```python
from build123d import *

# Parameters (mm, degrees)
SKETCH4_R             = 1.5
BOSS_EXTRUDE3_DEPTH   = 15
BOSS_EXTRUDE3_2_DEPTH = 15
BOSS_EXTRUDE3_3_DEPTH = 15
BOSS_EXTRUDE23_START  = 15
BOSS_EXTRUDE23_DEPTH  = 4
BOSS_EXTRUDE24_START  = 8
BOSS_EXTRUDE24_DEPTH  = 4
FILLET2_R             = 2
FILLET1_R             = 1.5


# Read off the part's stored shape, not the designer's step: Mirror15
with BuildPart() as part:
    # Sketch4 → Boss-Extrude3 (new, symmetric)
    with BuildSketch(Plane.XY):
        with BuildLine():
            ThreePointArc((-15.745615363, 108.217071894), (-14.863780591, 107.808507644), (-13.893474834, 107.863861505))
            ThreePointArc((-13.893474834, 107.863861505), (-10.727575159, 106.958592694), (-10.299299114, 103.693778456))
            ThreePointArc((-10.299299114, 103.693778456), (-11.193367854, 101.14903756), (-11.496495568, 98.468892279))
            Line((-11.496495568, 98.468892279), (-11.496495568, 91.5))
            Line((-11.496495568, 91.5), (-13, 90))
            Line((-13, 90), (-14.503504432, 90))
            Line((-14.503504432, 90), (-14.503504432, 95.734709942))
            ThreePointArc((-14.503504432, 95.734709942), (-17.04172216, 103.115406131), (-23.582617138, 107.373800002))
            ThreePointArc((-23.582617138, 107.373800002), (-29.032421023, 126.907705171), (-20.414545428, 145.265429262))
            ThreePointArc((-20.414545428, 145.265429262), (-19.127581616, 145.281958408), (-19.054880744, 143.996943368))
            ThreePointArc((-19.054880744, 143.996943368), (-24.95633052, 125.408148717), (-15.745615363, 108.217071894))
        make_face()
        with Locations((-13, 105)):
            Circle(SKETCH4_R, mode=Mode.SUBTRACT)
    extrude(amount=BOSS_EXTRUDE3_DEPTH, both=True)



with BuildPart() as body_2:
    # Sketch4 → Boss-Extrude3 2 (new, symmetric)
    with BuildSketch(Plane.XY):
        with BuildLine():
            ThreePointArc((-15.463298435, 144.692144482), (-19.624699769, 139.278232713), (-21.960734627, 132.861797344))
            ThreePointArc((-21.960734627, 132.861797344), (-20.98224362, 131.398279383), (-19.518725659, 132.37677039))
            ThreePointArc((-19.518725659, 132.37677039), (-17.442455247, 138.079705369), (-13.743797057, 142.891596244))
            ThreePointArc((-13.743797057, 142.891596244), (-13.703273627, 144.651621052), (-15.463298435, 144.692144482))
        make_face()
    extrude(amount=BOSS_EXTRUDE3_2_DEPTH, both=True)


with BuildPart() as body_3:
    # Sketch4 → Boss-Extrude3 3 (new, symmetric)
    with BuildSketch(Plane.XY):
        with BuildLine():
            ThreePointArc((-18.842097465, 122.098018813), (-15.492555186, 116.010374953), (-10.254266127, 111.445381089))
            ThreePointArc((-10.254266127, 111.445381089), (-9.828866365, 109.737058954), (-11.5371885, 109.311659193))
            ThreePointArc((-11.5371885, 109.311659193), (-17.430845593, 114.447784397), (-21.199452745, 121.297059992))
            ThreePointArc((-21.199452745, 121.297059992), (-20.421254515, 122.876217042), (-18.842097465, 122.098018813))
        make_face()
    extrude(amount=BOSS_EXTRUDE3_3_DEPTH, both=True)


with BuildPart() as part_1:
    add(part.part)

    add(body_2.part)  # Boss-Extrude23 merges body 2

    add(body_3.part)  # Boss-Extrude23 merges body 3
    # Sketch81 → Boss-Extrude23 (add)
    with BuildSketch(Plane.XY.offset(BOSS_EXTRUDE23_START)):
        with BuildLine():
            ThreePointArc((-16.40923932, 143.732728133), (-16.959334589, 143.117801193), (-17.486399904, 142.483023987))
            ThreePointArc((-17.486399904, 142.483023987), (-20.86751312, 139.665952099), (-23.582500348, 136.202331891))
            ThreePointArc((-23.582500348, 136.202331891), (-23.172403472, 137.265482274), (-22.71440592, 138.308893232))
            ThreePointArc((-22.71440592, 138.308893232), (-19.828313947, 141.330604813), (-16.40923932, 143.732728133))
        make_face()
        with BuildLine():
            ThreePointArc((-14.984055873, 111.863377416), (-19.218265584, 114.528225057), (-23.012819409, 117.788793427))
            ThreePointArc((-23.012819409, 117.788793427), (-22.730989821, 117.159440449), (-22.431952643, 116.538079158))
            ThreePointArc((-22.431952643, 116.538079158), (-18.094842505, 113.132119318), (-13.268041623, 110.465083507))
            ThreePointArc((-13.268041623, 110.465083507), (-14.143339764, 111.14301058), (-14.984055873, 111.863377416))
        make_face()
    extrude(amount=-BOSS_EXTRUDE23_DEPTH)

    # Sketch81<4> → Boss-Extrude24 (add)
    with BuildSketch(Plane.XY.offset(BOSS_EXTRUDE24_START)):
        with BuildLine():
            ThreePointArc((-20.65110959, 119.849519429), (-20.27231766, 118.99567056), (-19.858240545, 118.158364546))
            ThreePointArc((-19.858240545, 118.158364546), (-18.627716165, 113.52909009), (-16.787605108, 109.106606226))
            ThreePointArc((-16.787605108, 109.106606226), (-17.300236642, 109.582181696), (-17.799401283, 110.071873209))
            ThreePointArc((-17.799401283, 110.071873209), (-19.571385864, 114.859745334), (-20.65110959, 119.849519429))
        make_face()
        with BuildLine():
            ThreePointArc((-19.934917917, 142.906651174), (-21.099885834, 138.172303965), (-21.85680447, 133.355845939))
            ThreePointArc((-21.85680447, 133.355845939), (-21.435815653, 134.965674653), (-20.896432339, 136.539792094))
            ThreePointArc((-20.896432339, 136.539792094), (-20.121005018, 140.27470116), (-19.095815217, 143.948911161))
            ThreePointArc((-19.095815217, 143.948911161), (-19.522323343, 143.433381929), (-19.934917917, 142.906651174))
        make_face()
    extrude(amount=-BOSS_EXTRUDE24_DEPTH)

    # SurfaceCut2: cut with a surface, the side it looks to stays
    # 3DSketch1 → Surface-Fill1: a flat surface bounded by the sketch
    with BuildSketch(Plane(origin=(-13, 90, 15), x_dir=(0.2636894274940136, 0.964607633096421, 0), z_dir=(-0.8532247447444736, 0.2332413063570551, -0.4664826127141099)), mode=Mode.PRIVATE) as surface_fill1_1_region:
        Polygon((0, 0), (5.701800205, 0), (1.843369672, 2.261086868), align=None)
    surface_fill1_1 = surface_fill1_1_region.sketch.faces()[0]
    split(bisect_by=surface_fill1_1, keep=Keep.TOP)

    # Fillet2
    fillet2_edges = [part_1.edges().sort_by_distance(p)[0] for p in [
        (-11.496495568, 93.5, 14),
        (-12.248247784, 90.75, 14),
    ]]
    fillet(fillet2_edges, radius=FILLET2_R)

    # Fillet1
    # the kernel refuses this fillet: 1.5 mm, written as the material it takes off along each edge
    with BuildSketch(Plane(origin=(-14.503504432, 86.25, 15), x_dir=(1, 0, 0), z_dir=(0, 1, 0)), Plane(origin=(-14.503504432, 86.25, -15), x_dir=(0, 0, 1), z_dir=(0, 1, 0))) as fillet1_piece_1:
        with BuildLine():
            CenterArc((FILLET1_R, FILLET1_R), FILLET1_R, 180, 90)
            Line((0, FILLET1_R), (0, 0))
            Line((0, 0), (FILLET1_R, 0))
        make_face()
    extrude(amount=9.484709942, mode=Mode.SUBTRACT)
    with BuildSketch(Plane(origin=(-26.503504432, 95.734709942, 15), x_dir=(1, 0, 0), z_dir=(0, -1, 0))) as fillet1_piece_2:
        with BuildLine():
            CenterArc((12 + FILLET1_R, -FILLET1_R), FILLET1_R, 90, 90)
            Line((12, -FILLET1_R), (12, 0))
            Line((12, 0), (12 + FILLET1_R, 0))
        make_face()
    revolve(axis=Axis((-26.503504432, 95.734709942, 15), (0, 0, 1)), revolution_arc=93.822319642, mode=Mode.SUBTRACT)
    with BuildSketch(Plane(origin=(-26.503504432, 95.734709942, -15), x_dir=(1, 0, 0), z_dir=(0, -1, 0))) as fillet1_piece_3:
        with BuildLine():
            CenterArc((12 + FILLET1_R, FILLET1_R), FILLET1_R, 180, 90)
            Line((12 + FILLET1_R, 0), (12, 0))
            Line((12, 0), (12, FILLET1_R))
        make_face()
    revolve(axis=Axis((-26.503504432, 95.734709942, -15), (0, 0, 1)), revolution_arc=93.822319642, mode=Mode.SUBTRACT)

    # Mirror15
    split(bisect_by=Plane.XY, keep=Keep.TOP)

    # Mirror15 2: part across plane


with BuildPart() as part_2:
    add(part_1.part)
    add(part_1.part.mirror(Plane.XY))


solid = part_2.part
```
Geometry check sheet. Reference: the model listing, model coordinates, mm. A direction names the side the tool comes from. Coordinates: 2 decimals unless noted, no trailing zeros. Loops run counter-clockwise (first coordinate to the right, second up) from the corner with the lowest first, then second, coordinate; pieces in that order, holes last. Notation, with made-up numbers: (12.25, 67) - (28.25, 67) arc R14 cw to (28.25, 85) - close; hole circle Ø11 at (71.25, -22). An arc over 180 degrees is marked (long way). One line per item, written item: value. Start each with the question number.
(1) Cross-section at B-B on y = 115.5. Enter the section's corners in (x, z).
(2) Mould release check, pull along Z, two halves, no side actions. Record for faces 4 (the flat face through (-20.24, 140.54, 11)), 5 (the cylindrical face through (-12.21, 90.96, 13.78)), 6 (the cylindrical face through (-14.88, 107.81, -0.21)): released by +Z, released by -Z, zero draft, split by the parting line, or undercut.
(3) Cross-section at A-A on z = 6.5. Enter the section's corners in (x, y), plus the area to 3 significant figures.
(4) Tool access check on faces 1 (the cylindrical face through (-17.483, 138.005, -0.21)), 2 (the cylindrical face through (-29.055, 126.619, -0.21)), 3 (the flat face through (-20.24, 140.54, -11)). Record the directions out of +Z, -Z, +X, -X, +Y, -Y that give a thin tool (end or side, any length) a straight path to the whole face; none if there is none.
(5) Cross-section at C-C on y = 126. Enter the section's corners in (x, z).
(6) Material ranges on line 1 (Z direction, x = -18.25, y = 112); line 2 (Y direction, x = -13, z = 8); line 3 (Y direction, x = -18.25, z = -3), recorded low to high. Write a range as [from, to].
(7) Depth check by flat-ended pin: P1, Ø1.5, axis at y = 105, z = -4.5, coming from the -X side; P2, Ø4.5, axis at y = 92, z = 9, coming from the -X side; P3, Ø4, axis at x = -27, z = -3.5, coming from the -Y side. Enter the tip coordinate at first touch or a pass-through.
(8) Cross-section at D-D on x = -28. Enter the section's corners in (y, z), plus the area to 3 significant figures.
Results below:
1. outline: (-27.72, -15) - (-21.88, -15) - (-21.88, 15) - (-27.72, 15) - close; (-21.26, -15) - (-20.47, -15) - (-20.47, -11) - (-21.26, -11) - close; (-21.26, 11) - (-20.47, 11) - (-20.47, 15) - (-21.26, 15) - close; (-19.75, -8) - (-19.23, -8) - (-19.23, -4) - (-19.75, -4) - close; (-19.75, 4) - (-19.23, 4) - (-19.23, 8) - (-19.75, 8) - close; (-18.23, -15) - (-15.07, -15) - (-15.07, 15) - (-18.23, 15) - close
2. face 4: undercut
2. face 5: released by +Z
2. face 6: zero draft
3. outline: (-23.58, 107.37) arc R12 cw to (-14.5, 95.73) - (-14.5, 90) - (-13, 90) - (-11.5, 91.5) - (-11.5, 98.47) arc R12 cw to (-10.3, 103.69) arc R3 ccw to (-13.89, 107.86) arc R2 cw to (-15.75, 108.22) arc R25.06 cw to (-16.79, 109.11) arc R35.64 cw to (-19.86, 118.16) arc R22.39 ccw to (-11.54, 109.31) arc R1.24 ccw to (-10.25, 111.45) arc R19.9 cw to (-18.84, 122.1) arc R1.24 ccw to (-21.2, 121.3) arc R22.39 ccw to (-20.65, 119.85) arc R36.14 ccw to (-17.8, 110.07) arc R25.06 cw to (-19.93, 142.91) arc R57.11 ccw to (-21.86, 133.36) arc R22.39 ccw to (-21.96, 132.86) arc R1.24 ccw to (-19.52, 132.38) arc R19.9 cw to (-13.74, 142.89) arc R1.24 ccw to (-15.46, 144.69) arc R22.39 ccw to (-20.9, 136.54) arc R56.61 cw to (-19.1, 143.95) arc R25.06 cw to (-19.05, 144) arc R0.93 ccw to (-20.41, 145.27) arc R29.13 ccw to start; hole circle Ø3 at (-13, 105)
3. area: 338 mm2
4. face 1: +Z, -Z, +X
4. face 2: +Z, -Z, -X
4. face 3: none
5. outline: (-29.09, -15) - (-25, -15) - (-25, 15) - (-29.09, 15) - close
6. line 1: z = [-8, -4], [4, 8]
6. line 2: y = [90, 103.5], [106.5, 108], [110.27, 113.43]
6. line 3: y = [104.45, 110.54], [115.53, 120.57], [136.43, 141.47]
7. P1: stops at x = -19.89
7. P2: stops at x = -14.5
7. P3: stops at y = 109.52
8. outline: (116.43, -15) - (132.53, -15) - (132.53, 15) - (116.43, 15) - close
8. area: 483 mm2
